Answer from the drawing. Dimensions are ordinates in mm from the lowest x, y and z of the part. A direction names the side the tool comes from. Give positions to 0.01 mm unless a question says otherwise; leave off trailing zeros. Loops run counter-clockwise (first coordinate to the right, second up) from the corner with the lowest first, then second, coordinate; pieces in that order, holes last. Notation, with made-up numbers: (59.25, 51.25) - (110.25, 51.25) arc R30 cw to (110.25, 74.25) - close; hole circle Ø3 at (74.5, 70). An arc over 180 degrees is marked (long way). One line per question, with ' | ' between items. Start each with the question number.
1. Find the intervals of material crossed by line 1 (Z direction, x = 8.5, y = 9); line 2 (Y direction, x = 31, z = 15); line 3 (Y direction, x = 11, z = 25.5), in increasing order.
2. For a pull along Z with two mould halves and no side action, classify the marked faces 1, 2, 3 and 4 as released by +Z, released by -Z, zero draft, split by the parting line, or undercut.
3. Section D-D (z = 32) is taken. Determine the outline of the cut face in (x, y).
4. Each of these flat-tipped pins is pushed along its axis until it touches: pin 1 (5 mm diameter, centred on x = 5, z = 77, fed in from +Y); pin 2 (10.5 mm diameter, centred on x = 19.5, z = 20, fed in from -Y); pin 3 (6 mm diameter, centred on x = 26, y = 19.5, fed in from -Z); pin 4 (2 mm diameter, centred on y = 19, z = 22.5, fed in from +X). Where does it stop, or does it pass through?
5. Section C-C (x = 2.5) is taken. Determine the outline of the cut face in (y, z).
6. Which of the six approach directions +Z, -Z, +X, -X, +Y, -Y give full straight-line access (tool end or side, diameter ignored) to the marked faces 5, 6, 7, 8 and 9?
7. Section A-A (y = 14) is taken. Determine the outline of the cut face in (x, z).
8. Section B-B (z = 80.5) is taken. Determine the outline of the cut face in (x, y).
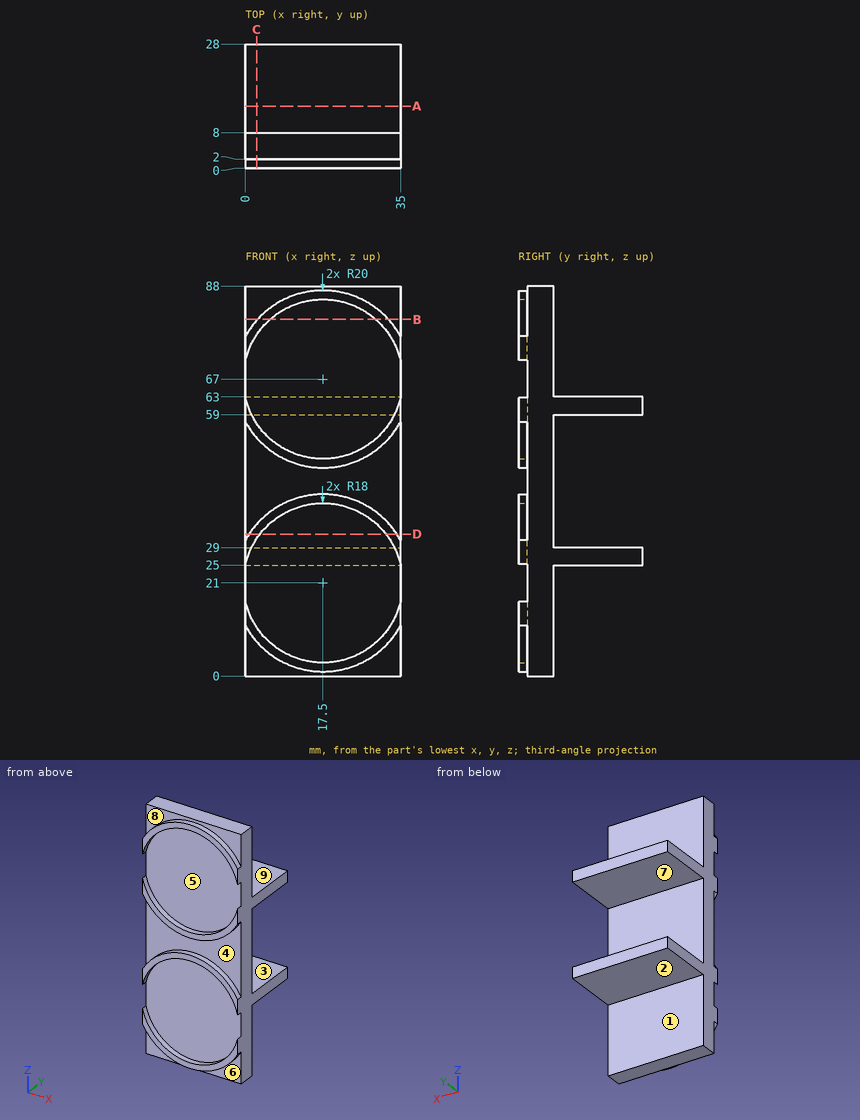
Conclusion:
1) line 1: 25 to 29, 59 to 63 | line 2: 2 to 8 | line 3: 2 to 28
2) face 1: zero draft | face 2: released by -Z | face 3: undercut | face 4: undercut
3) outline: (0, 2) - (0.8, 2) - (0.8, 0) - (3.25, 0) - (3.25, 2) - (31.75, 2) - (31.75, 0) - (34.2, 0) - (34.2, 2) - (35, 2) - (35, 8) - (0, 8) - close
4) pin 1: y = 8 | pin 2: y = 2 | pin 3: z = 25 | pin 4: through
5) outline: (0, 7.77) - (2, 7.77) - (2, 0) - (8, 0) - (8, 25) - (28, 25) - (28, 29) - (8, 29) - (8, 59) - (28, 59) - (28, 63) - (8, 63) - (8, 88) - (2, 88) - (2, 80.23) - (0, 80.23) - (0, 76.95) - (2, 76.95) - (2, 57.05) - (0, 57.05) - (0, 53.77) - (2, 53.77) - (2, 34.23) - (0, 34.23) - (0, 30.95) - (2, 30.95) - (2, 11.05) - (0, 11.05) - close
6) face 5: -Y | face 6: -Z, -Y | face 7: +X, -X, +Y | face 8: +Z, -Y | face 9: +Z, +X, -X, +Y
7) outline: (0, 25) - (35, 25) - (35, 29) - (0, 29) - close; (0, 59) - (35, 59) - (35, 63) - (0, 63) - close
8) outline: (0, 2) - (2.74, 2) - (2.74, 0) - (5.59, 0) - (5.59, 2) - (29.41, 2) - (29.41, 0) - (32.26, 0) - (32.26, 2) - (35, 2) - (35, 8) - (0, 8) - close
